Input: dimensioned drawing with shaded views. Units: mm. Origin: part minimum x, y, z. Give positions to 0.01 mm unless a question says otherwise; leave off trailing zeros. Write each loop counter-clockwise with the first axis right and the second up, starting at its lowest first coordinate (ties: lowest second). Pieces come first, ordered by that corner, then holes.
Q1. Section C-C (y = 6). State how many separate pieces and enclosed holes the cut face has, plus the area to 3 significant figures.
Q2. Section B-B (z = 34). Return the cut outline in (x, y), plus the area to 3 significant figures.
Q3. Line query: line 1 (Z direction, x = 8, y = 1.5); line 2 (Z direction, x = 27.5, y = 6). Output: solid intervals per line, ascending.
Q4. Section A-A (x = 18). Return the cut outline in (y, z), plus the area to 3 significant figures.
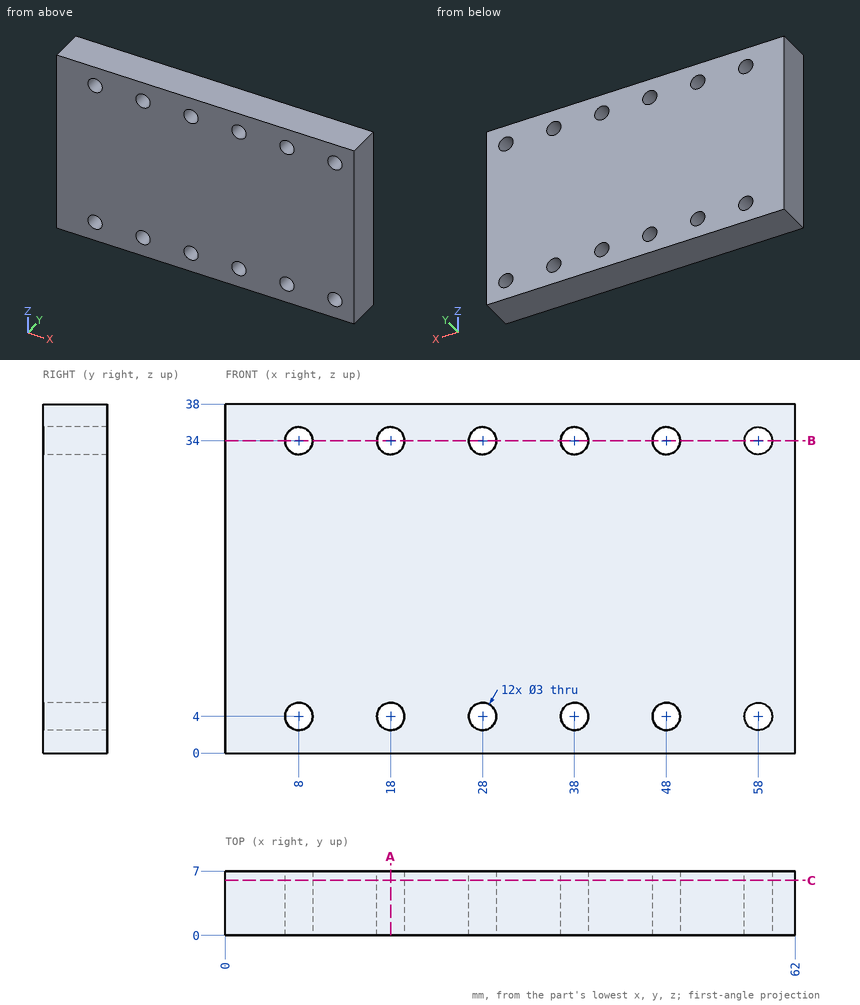
Computed:
1. separate pieces: 1
1. enclosed holes: 12
1. area: 2,270 mm2
2. outline: (0, 0) - (6.5, 0) - (6.5, 7) - (0, 7) - close; (9.5, 0) - (16.5, 0) - (16.5, 7) - (9.5, 7) - close; (19.5, 0) - (26.5, 0) - (26.5, 7) - (19.5, 7) - close; (29.5, 0) - (36.5, 0) - (36.5, 7) - (29.5, 7) - close; (39.5, 0) - (46.5, 0) - (46.5, 7) - (39.5, 7) - close; (49.5, 0) - (56.5, 0) - (56.5, 7) - (49.5, 7) - close; (59.5, 0) - (62, 0) - (62, 7) - (59.5, 7) - close
2. area: 308 mm2
3. line 1: z = 0 to 2.5, 5.5 to 32.5, 35.5 to 38
3. line 2: z = 0 to 2.59, 5.41 to 32.59, 35.41 to 38
4. outline: (0, 0) - (7, 0) - (7, 2.5) - (0, 2.5) - close; (0, 5.5) - (7, 5.5) - (7, 32.5) - (0, 32.5) - close; (0, 35.5) - (7, 35.5) - (7, 38) - (0, 38) - close
4. area: 224 mm2
